Study the drawing (mm; zero at the part's minimum x, y, z) and answer. A direction names the side the tool comes from. Round coordinates to 2 decimals unless told otherwise and drop trailing zeros. Loops run counter-clockwise (first coordinate to the right, second up) from the corner with the lowest first, then second, coordinate; pieces in that order, holes last. Notation, with made-up numbers: M 33,-17.5 L 72,-17.5 A7 ccw 72,-4.5 Z; hole C 53.25,77.25 d8. An arc over 180 degrees is marked long. Write each question's results on one line, items separated by ' | '.
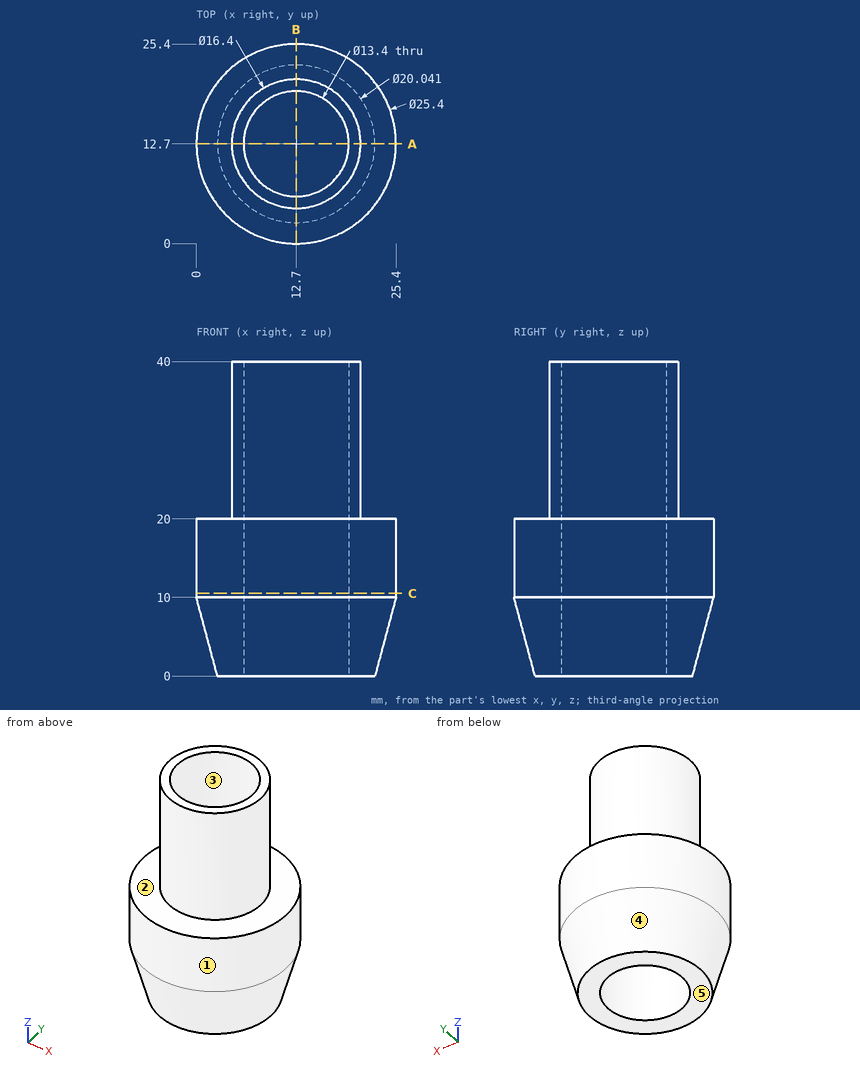
Item 1: Flat-ended cylindrical pins translate along their axes: pin 1 (5 mm diameter, centred on x = 6, z = 26.5, fed in from +Y); pin 2 (5 mm diameter, centred on y = 19, z = 11.5, fed in from +X); pin 3 (1 mm diameter, centred on x = 15.5, z = 11, fed in from +Y); pin 4 (5 mm diameter, centred on x = 4.5, y = 15, fed in from -Z). Find the tip coordinate at first contact, or state that the pin passes through.
Outcome:
pin 1: stops at y = 19.74 | pin 2: stops at x = 24.82 | pin 3: stops at y = 25.19 | pin 4: stops at z = 0
Item 2: Straight lines are drawn through the part: line 1 (Y direction, x = 12.7, z = 28); line 2 (Y direction, x = 12.7, z = 19.5); line 3 (X direction, y = 8.5, z = 26). For each, find the intervals that lie inside material, in ascending order.
Outcome:
line 1: y = 4.5 to 6, 19.4 to 20.9 | line 2: y = 0 to 6, 19.4 to 25.4 | line 3: x = 5.66 to 7.48, 17.92 to 19.74
Item 3: The mould has two halves that part along X. Classify the marked faces 3, 4 and 5: pulls with the +X half, pulls with the -X half, needs draft (parallel to the pull), parting line crosses it, or undercut.
Outcome:
face 3: undercut | face 4: parting line crosses it | face 5: needs draft
Item 4: The part is cut by section A-A (y = 12.7). Determine the outline of the cut face in (x, z), plus the area to 3 significant figures.
Outcome:
outline: M 0,10 L 2.68,0 L 6,0 L 6,40 L 4.5,40 L 4.5,20 L 0,20 Z; M 19.4,0 L 22.72,0 L 25.4,10 L 25.4,20 L 20.9,20 L 20.9,40 L 19.4,40 Z | area: 273 mm2
Item 5: The part is cut by section C-C (z = 10.5). Determine the outline of the cut face in (x, y), plus the area to 3 significant figures.
Outcome:
outline: C 12.7,12.7 d25.4; hole C 12.7,12.7 d13.4 | area: 366 mm2
Item 6: For the marked faces 1 and 2, determine the directions among +Z, -Z, +X, -X, +Y, -Y from which every point of the face is accessible in a straight line to the end or side of a thin tool.
Outcome:
face 1: +Z, -Z | face 2: +Z
